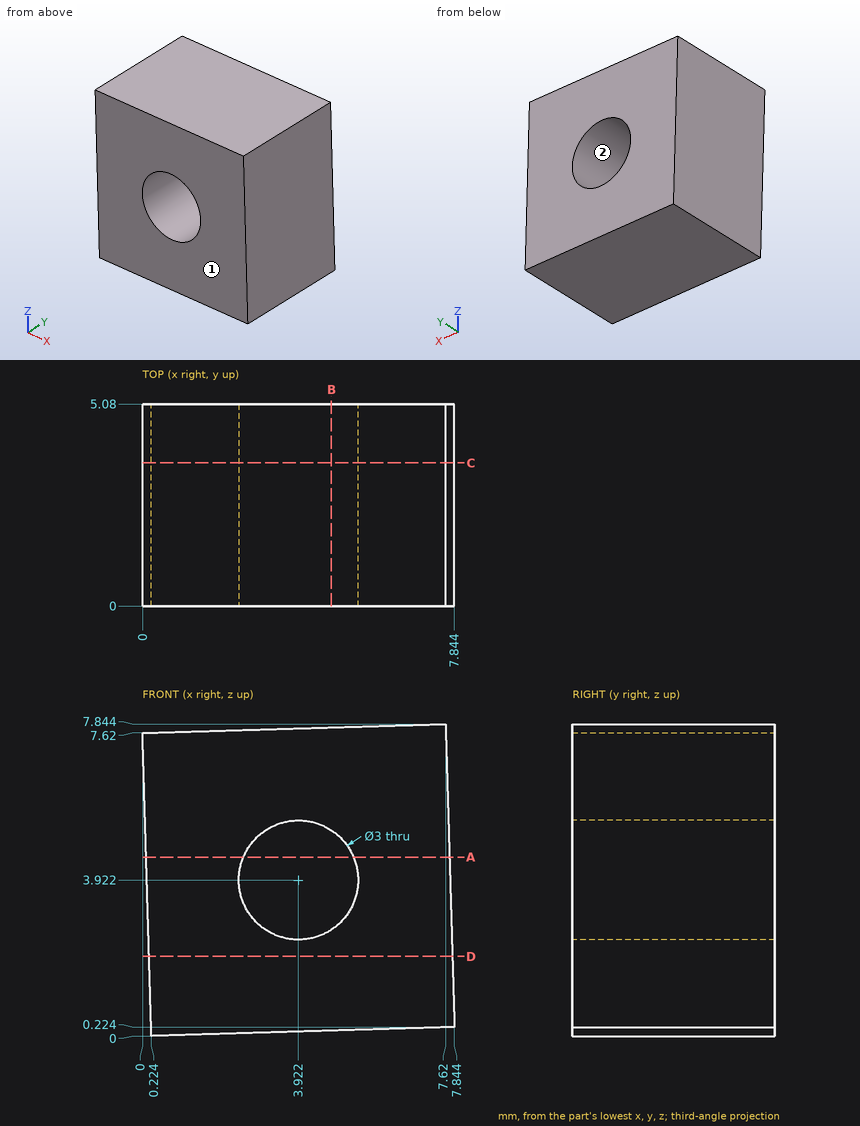
The figure shows three views and two pictorial views of one solid part (mm, origin at its lowest corner). Answer the questions. Round coordinates to 2 decimals unless told otherwise and drop trailing zeros. Order: outer loops, then holes, each group sorted by start corner. A loop starts at its lowest first (then second) coordinate and runs counter-clockwise, first axis right, second up. Notation, with made-up numbers: (44, 1) - (83, 1) arc R17 ccw to (83, 31) - close; hole circle Ø9 at (8, 31.25). An arc over 180 degrees is marked (long way). Write item = value, one per line. Start each with the question number.
1) Section B-B, the plane x = 4.75 is taken. Write down the section's boundary in (y, z).
2) Straight lines are drawn through the part: L1, parallel to X at y = 3, z = 5 (1 decimal); L2, parallel to Z at x = 3.25, y = 1.3 (1 decimal); L3, parallel to Z at x = 4, y = 2.4. For each, find the intervals that lie inside material, in ascending order.
3) Given pin 1 (3 mm diameter, centred on x = 2, y = 2.5, fed in from +Z), flat-ended and moving along its own axis, determine where the tip first touches the part or whether it passes through.
4) Section C-C, the plane y = 3.6 is taken. Write down the section's boundary in (x, z).
5) Section D-D, the plane z = 2 is taken. Write down the section's boundary in (x, y) (1 decimal).
6) Section A-A, the plane z = 4.5 is taken. Write down the section's boundary in (x, y), plus the area to 3 significant figures.
7) For a pull along X with two mould halves and no side action, classify the marked faces 1 and 2 as released by +X, released by -X, zero draft, split by the parting line, or undercut.
Results list:
q1.outline = (0, 0.13) - (5.08, 0.13) - (5.08, 2.67) - (0, 2.67) - close; (0, 5.17) - (5.08, 5.17) - (5.08, 7.76) - (0, 7.76) - close
q2.L1 = 0.1 to 2.9, 5 to 7.7
q2.L2 = 0.1 to 2.6, 5.3 to 7.7
q2.L3 = 0.11 to 2.42, 5.42 to 7.74
q3.pin_1 = 7.72
q4.outline = (0, 7.62) - (0.22, 0) - (7.84, 0.22) - (7.62, 7.84) - close; hole circle Ø3 at (3.92, 3.92)
q5.outline = (0.2, 0) - (7.8, 0) - (7.8, 5.1) - (0.2, 5.1) - close
q6.outline = (0.09, 0) - (2.54, 0) - (2.54, 5.08) - (0.09, 5.08) - close; (5.31, 0) - (7.72, 0) - (7.72, 5.08) - (5.31, 5.08) - close
q6.area = 24.7 mm^2
q7.face_1 = zero draft
q7.face_2 = undercut
